Check sheet for the modelled part. Datum: model origin and axes. Units: mm. Face numbers are marked on the shaded views. Coordinates: 2 decimals unless noted, no trailing zeros. Write each loop counter-clockwise with the first axis right and the second up, starting at its lowest first coordinate (ties: lowest second). Pieces come first, ordered by that corner, then holes. Notation, with made-up numbers: (52.25, -25.75) -> (80.25, -25.75) arc R33 cw to (80.25, 10.25) -> close; hole circle Ø6 at (-22, 46). An arc over 180 degrees is marked (long way). One line per item, written item: value. Start each with the question number.
1) Sectioned sample at A-A on z = 0.95. Enter the section's corners in (x, y), plus the area to 3 significant figures.
2) Draft check along X on the marked faces 1 and 2. Enter one of: +X half, -X half, draft (parallel to the pull), parting line (faces both ways), or undercut.
3) Gauge pin test, flat end, axial feed: P1, Ø0.5, axis at y = -0.5, z = 1, coming from the -X side. Record the tip position at first contact, or that the pin passes through.
4) Sectioned sample at B-B on x = 26. Enter the section's corners in (y, z), plus the area to 3 significant figures.
5) Scan lines: line 1 along Y through (x, z) = (25.75, 0.35); line 2 along X through (y, z) = (-0.25, 1.4); line 3 along Y through (x, z) = (28.25, 1.05). Record each from-to range of solid material in increasing order. Write a range as [from, to].
6) Sectioned sample at D-D on x = 16.5. Enter the section's corners in (y, z), plus the area to 3 significant figures.
7) Sectioned sample at C-C on y = -2. Enter the section's corners in (x, z).
```python
from build123d import *

# Parameters (mm, degrees)
BOSS_EXTRUDE1_DEPTH = 1.524


with BuildPart() as part:
    # Sketch1 → Boss-Extrude1 (new body)
    with BuildSketch(Plane.XY):
        with BuildLine():
            Line((4.36034561, 0), (4.36034561, -1.524))
            Line((4.36034561, -1.524), (-0.270041396, -1.524))
            ThreePointArc((-0.270041396, -1.524), (5.57790397, -4.249042789), (11.964164328, -5.165558929))
            ThreePointArc((11.964164328, -5.165558929), (12.599243088, -5.082111381), (13.193252116, -4.842441192))
            ThreePointArc((13.193252116, -4.842441192), (18.3130715, -2.621767508), (23.773581772, -1.469912607))
            ThreePointArc((23.773581772, -1.469912607), (26.795642109, -1.350433231), (29.50183022, 0))
            Line((29.50183022, 0), (29.028606423, 1.061962035))
            Line((29.028606423, 1.061962035), (25.453006053, -0.002386196))
            ThreePointArc((25.453006053, -0.002386196), (23.593059825, 0.239006946), (25.018211481, 1.458274504))
            Line((25.018211481, 1.458274504), (28.403024501, 2.465831103))
            Line((28.403024501, 2.465831103), (27.891133112, 3.614567125))
            ThreePointArc((27.891133112, 3.614567125), (17.871956928, 1.891446971), (8.033839359, 4.453570535))
            ThreePointArc((8.033839359, 4.453570535), (3.185317895, 3.52559175), (-0.270041396, 0))
            Line((-0.270041396, 0), (4.36034561, 0))
        make_face()
    extrude(amount=BOSS_EXTRUDE1_DEPTH)


solid = part.part
```
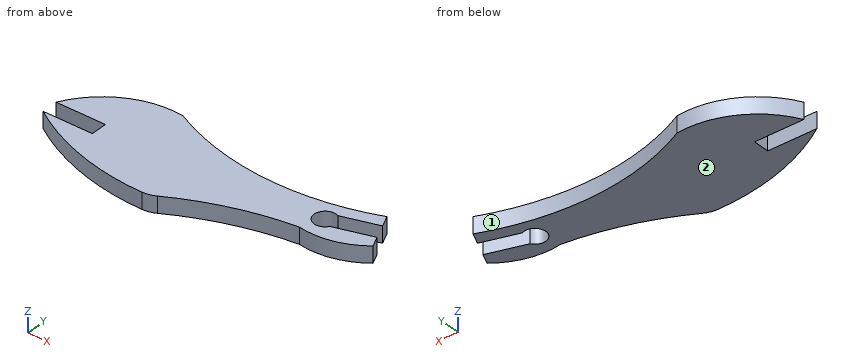
Answers:
1. outline: (-0.27, -1.52) arc R22.06 ccw to (11.96, -5.17) arc R2.54 ccw to (13.19, -4.84) arc R27.76 cw to (23.77, -1.47) arc R7.2 ccw to (29.5, 0) -> (29.03, 1.06) -> (25.45, 0) arc R1.03 cw (long way) to (25.02, 1.46) -> (28.4, 2.47) -> (27.89, 3.61) arc R24.1 cw to (8.03, 4.45) arc R8.27 ccw to (-0.27, 0) -> (4.36, 0) -> (4.36, -1.52) -> close
1. area: 158 mm2
2. face 1: undercut
2. face 2: draft
3. P1: stops at x = 4.36
4. outline: (-1.51, 0) -> (0.16, 0) -> (0.16, 1.52) -> (-1.51, 1.52) -> close; (1.75, 0) -> (2.94, 0) -> (2.94, 1.52) -> (1.75, 1.52) -> close
4. area: 4.36 mm2
5. line 1: y = [-1.54, 0.09], [1.68, 2.87]
5. line 2: x = [4.36, 23.91], [25.24, 29.17]
5. line 3: y = [-0.8, 0.83], [2.42, 2.81]
6. outline: (-3.27, 0) -> (1.99, 0) -> (1.99, 1.52) -> (-3.27, 1.52) -> close
6. area: 8.01 mm2
7. outline: (0.48, 0) -> (20.6, 0) -> (20.6, 1.52) -> (0.48, 1.52) -> close
